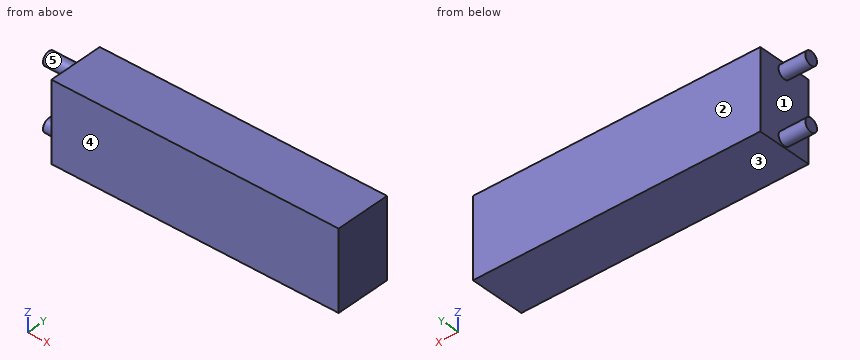
```python
from build123d import *

# Parameters (mm, degrees)
SKETCH1_W           = 64.5
SKETCH1_H           = 17.7
BOSS_EXTRUDE1_DEPTH = 6.2
SKETCH2_R           = 1.5
BOSS_EXTRUDE2_DEPTH = 6


with BuildPart() as part:
    # Sketch1 → Boss-Extrude1 (new, symmetric)
    with BuildSketch(Plane(origin=(0, 0, 0), x_dir=(1, 0, 0), z_dir=(0, 1, 0))):
        Rectangle(SKETCH1_W, SKETCH1_H)
    extrude(amount=BOSS_EXTRUDE1_DEPTH, both=True)

    # Sketch2 → Boss-Extrude2 (add, symmetric)
    with BuildSketch(Plane.ZY.offset(32.25)):
        with Locations(Location((-7, 0, 0), (0, 0, 180))):
            Circle(SKETCH2_R)
        with Locations(Location((7, 0, 0), (0, 0, 180))):
            Circle(SKETCH2_R)
    extrude(amount=BOSS_EXTRUDE2_DEPTH, both=True)


solid = part.part
```
Design review of the part built by this model. Coordinates are the model's own, in mm. Face numbers are marked on the shaded views. A direction names the side the tool comes from. Give positions to 0.01 mm unless a question says otherwise; leave off trailing zeros. Order: outer loops, then holes, each group sorted by start corner. A loop starts at its lowest first (then second) coordinate and runs counter-clockwise, first axis right, second up. Notation, with made-up numbers: (82.5, 16.25) -> (139.5, 16.25) arc R10 ccw to (139.5, 27.25) -> close; hole circle Ø6 at (12, 40.25). An arc over 180 degrees is marked (long way). Write item = value, one per line. Start each with the question number.
(1) We need section C-C on z = 1. Write out the cut boundary in (x, y), plus the area to 3 significant figures.
(2) Mouldability with a two-part tool opening along Z and no side actions: class the marked faces 3, 4 and 5 as +Z half, -Z half, draft (parallel to the pull), parting line (faces both ways), or undercut.
(3) For the marked faces 1 and 2, list the 3-axis set-ups (+Z, -Z, +X, -X, +Y, -Y) from which the entire face can be reached by the end or side of a thin tool; tool diameter is ignored.
(4) We need section D-D on y = 4. Write out the cut boundary in (x, z), plus the area to 3 significant figures.
(5) To check wall thickness, follow line 1 along X through (y, z) = (1.25, 1). State the ranges of the line that lie inside material, in increasing order.
(6) We need section A-A on y = 0. Write out the cut boundary in (x, z).
(7) We need section B-B on z = -7. Write out the cut boundary in (x, y), plus the area to 3 significant figures.
(8) For pin 1 (3 mm diameter, centred on y = 3, z = -5.5, fed in from -X), flat-tipped, find the tip position at first contact; note if it passes through.
Numbers:
q1.outline = (-32.25, -6.2) -> (32.25, -6.2) -> (32.25, 6.2) -> (-32.25, 6.2) -> close
q1.area = 800 mm^2
q2.face_3 = -Z half
q2.face_4 = draft
q2.face_5 = undercut
q3.face_1 = -X
q3.face_2 = +Z, -Z, +X, -X, +Y
q4.outline = (-32.25, -8.85) -> (32.25, -8.85) -> (32.25, 8.85) -> (-32.25, 8.85) -> close
q4.area = 1,140 mm^2
q5.line_1 = -32.25 to 32.25
q6.outline = (-38.25, -8.5) -> (-32.25, -8.5) -> (-32.25, -8.85) -> (32.25, -8.85) -> (32.25, 8.85) -> (-32.25, 8.85) -> (-32.25, 8.5) -> (-38.25, 8.5) -> (-38.25, 5.5) -> (-32.25, 5.5) -> (-32.25, -5.5) -> (-38.25, -5.5) -> close
q7.outline = (-38.25, -1.5) -> (-32.25, -1.5) -> (-32.25, -6.2) -> (32.25, -6.2) -> (32.25, 6.2) -> (-32.25, 6.2) -> (-32.25, 1.5) -> (-38.25, 1.5) -> close
q7.area = 818 mm^2
q8.pin_1 = -32.25
